from build123d import *

# Parameters (mm, degrees)
SKETCH_1_W          = 15
SKETCH_1_H          = 15
SKETCH_1_W_2        = 13
SKETCH_1_H_2        = 13
EXTRUDE_1_DEPTH     = 180
SKETCH_2_R          = 1.45
CUT_EXTRUDE_1_DEPTH = 181.779561898
SKETCH_3_R          = 1.45
CUT_EXTRUDE_2_DEPTH = 181.779561898


with BuildPart() as part:
    # 草图1 → 凸台-拉伸1 (new body)
    with BuildSketch(Plane(origin=(0, 0, 0), x_dir=(0, 0, -1), z_dir=(1, 0, 0))):
        Rectangle(SKETCH_1_W, SKETCH_1_H)
        Rectangle(SKETCH_1_W_2, SKETCH_1_H_2, mode=Mode.SUBTRACT)
    extrude(amount=EXTRUDE_1_DEPTH)

    # 草图2 → 切除-拉伸1 (cut, through all)
    with BuildSketch(Plane(origin=(0, 7.5, 0), x_dir=(1, 0, 0), z_dir=(0, 1, 0))):
        with Locations(Location((10, 0, 0), (0, 0, 270))):
            Circle(SKETCH_2_R)
        with Locations(Location((170, 0, 0), (0, 0, 270))):
            Circle(SKETCH_2_R)
    extrude(amount=-CUT_EXTRUDE_1_DEPTH, mode=Mode.SUBTRACT)

    # 草图3 → 切除-拉伸2 (cut, through all)
    with BuildSketch(Plane.XY.offset(7.5)):
        with Locations((15, 0)):
            Circle(SKETCH_3_R)
        with Locations((165, 0)):
            Circle(SKETCH_3_R)
    extrude(amount=-CUT_EXTRUDE_2_DEPTH, mode=Mode.SUBTRACT)


solid = part.part
Geometry: final body of the model. Coordinates: model frame, mm. A direction names the side the tool comes from. Coordinates: 2 decimals unless noted, no trailing zeros. Order: outer loops, then holes, each group sorted by start corner. A loop starts at its lowest first (then second) coordinate and runs counter-clockwise, first axis right, second up.
(1) Section query A-A (x = 40). Return the cut outline in (y, z).
(2) Draft query along X for faces 3 (the face through (166.38, 0.44, -6.99)), 4 (the face through (0, 0, 7)), 5 (the face through (180, 0, 7)), 6 (the face through (89, 6.5, 0)). Return one class per face: pulls with the +X half, pulls with the -X half, needs draft (parallel to the pull), parting line crosses it, or undercut.
(3) First-contact query: pin 1 (2.5 mm diameter, centred on x = 15, y = 0, fed in from +Z). Flat tip, straight axial feed; report the tip coordinate or a pass-through.
(4) Access query for faces 1 (the face through (89, 0, 6.5)), 2 (the face through (16.38, 0.44, 7.01)). Directions: +Z, -Z, +X, -X, +Y, -Y. A direction counts if a zero-diameter tool reaches every point of the face in a straight line with its end or side. Return the directions, or none.
(5) Section query B-B (z = 0). Return the cut outline in (x, y), plus the area to 3 significant figures.
(6) Section query C-C (y = 0). Return the cut outline in (x, z).
(7) Section query D-D (x = 15). Return the cut outline in (y, z), plus the area to 3 significant figures.
(8) Material intervals for probe 1 along X at (y, z) = (7.3, 0); probe 2 along Z at (x, y) = (170, 7.35); probe 3 along Y at (x, z) = (60, -4), sorted ascending.
Solution:
1. outline: (-7.5, -7.5) - (7.5, -7.5) - (7.5, 7.5) - (-7.5, 7.5) - close; hole (-6.5, -6.5) - (6.5, -6.5) - (6.5, 6.5) - (-6.5, 6.5) - close
2. face 3: undercut
2. face 4: pulls with the -X half
2. face 5: pulls with the +X half
2. face 6: needs draft
3. pin 1: passes through
4. face 1: +X, -X
4. face 2: +Z, -Z
5. outline: (0, -7.5) - (8.55, -7.5) - (8.55, -6.5) - (0, -6.5) - close; (0, 6.5) - (8.55, 6.5) - (8.55, 7.5) - (0, 7.5) - close; (11.45, -7.5) - (168.55, -7.5) - (168.55, -6.5) - (11.45, -6.5) - close; (11.45, 6.5) - (168.55, 6.5) - (168.55, 7.5) - (11.45, 7.5) - close; (171.45, -7.5) - (180, -7.5) - (180, -6.5) - (171.45, -6.5) - close; (171.45, 6.5) - (180, 6.5) - (180, 7.5) - (171.45, 7.5) - close
5. area: 348 mm2
6. outline: (0, -7.5) - (13.55, -7.5) - (13.55, -6.5) - (0, -6.5) - close; (0, 6.5) - (13.55, 6.5) - (13.55, 7.5) - (0, 7.5) - close; (16.45, -7.5) - (163.55, -7.5) - (163.55, -6.5) - (16.45, -6.5) - close; (16.45, 6.5) - (163.55, 6.5) - (163.55, 7.5) - (16.45, 7.5) - close; (166.45, -7.5) - (180, -7.5) - (180, -6.5) - (166.45, -6.5) - close; (166.45, 6.5) - (180, 6.5) - (180, 7.5) - (166.45, 7.5) - close
7. outline: (-7.5, -7.5) - (-1.45, -7.5) - (-1.45, -6.5) - (-6.5, -6.5) - (-6.5, 6.5) - (-1.45, 6.5) - (-1.45, 7.5) - (-7.5, 7.5) - close; (1.45, -7.5) - (7.5, -7.5) - (7.5, 7.5) - (1.45, 7.5) - (1.45, 6.5) - (6.5, 6.5) - (6.5, -6.5) - (1.45, -6.5) - close
7. area: 50.2 mm2
8. probe 1: x = 0 to 8.55, 11.45 to 168.55, 171.45 to 180
8. probe 2: z = -7.5 to -1.45, 1.45 to 7.5
8. probe 3: y = -7.5 to -6.5, 6.5 to 7.5
